from build123d import *

# Parameters (mm, degrees)
BOSS_EXTRUDE1_DEPTH      = 2
SKETCH3_R                = 0.5
CUT_EXTRUDE1_DEPTH       = 2
SKETCH4_R                = 0.75
BOSS_EXTRUDE2_DEPTH      = 1
SKETCH5_R                = 0.5
CUT_EXTRUDE2_DEPTH       = 2
BOSS_EXTRUDE3_DEPTH      = 3
BOSS_EXTRUDE3_DEPTH_BACK = 6
SKETCH6_R                = 2.5
SKETCH7_R                = 0.75
BOSS_EXTRUDE4_DEPTH      = 5
SKETCH9_R                = 0.65
BOSS_EXTRUDE5_DEPTH      = 0.3
BOSS_EXTRUDE6_DEPTH      = 2


with BuildPart() as part:
    # Sketch2 → Boss-Extrude1 (new body)
    with BuildSketch(Plane.XY):
        with BuildLine():
            Line((-7.9375, -2.462871108), (-7.9375, 2.462871108))
            ThreePointArc((-7.9375, 2.462871108), (-7.792847338, 2.889004109), (-7.418673332, 3.139019187))
            Line((-7.418673332, 3.139019187), (-0.924016143, 4.879257336))
            Line((-0.924016143, 4.879257336), (3.375983857, 4.879257336))
            ThreePointArc((3.375983857, 4.879257336), (3.870958604, 4.674232083), (4.075983857, 4.179257336))
            Line((4.075983857, 4.179257336), (4.075983857, 2.879257336))
            Line((4.075983857, 2.879257336), (7.075983857, 2.879257336))
            Line((7.075983857, 2.879257336), (7.075983857, 3.545029821))
            ThreePointArc((7.075983857, 3.545029821), (7.326032531, 4.081260931), (7.897537582, 4.234395248))
            Line((7.897537582, 4.234395248), (11.484053724, 3.601995685))
            ThreePointArc((11.484053724, 3.601995685), (11.89873111, 3.362581585), (12.0625, 2.912630258))
            Line((12.0625, 2.912630258), (12.0625, -2.912630258))
            ThreePointArc((12.0625, -2.912630258), (11.89873111, -3.362581585), (11.484053724, -3.601995685))
            Line((11.484053724, -3.601995685), (7.897537582, -4.234395248))
            ThreePointArc((7.897537582, -4.234395248), (7.326032531, -4.081260931), (7.075983857, -3.545029821))
            Line((7.075983857, -3.545029821), (7.075983857, -2.879257336))
            Line((7.075983857, -2.879257336), (4.075983857, -2.879257336))
            Line((4.075983857, -2.879257336), (4.075983857, -4.179257336))
            ThreePointArc((4.075983857, -4.179257336), (3.870958604, -4.674232083), (3.375983857, -4.879257336))
            Line((3.375983857, -4.879257336), (-0.924016143, -4.879257336))
            Line((-0.924016143, -4.879257336), (-7.418673332, -3.139019187))
            ThreePointArc((-7.418673332, -3.139019187), (-7.792847338, -2.889004109), (-7.9375, -2.462871108))
        make_face()
    extrude(amount=BOSS_EXTRUDE1_DEPTH)

    # Sketch3 → Cut-Extrude1 (cut)
    with BuildSketch(Plane.XY.offset(2)):
        with Locations((8.575983857, 2.879257336)):
            Circle(SKETCH3_R)
        with Locations((8.575983857, -2.879257336)):
            Circle(SKETCH3_R)
    extrude(amount=-CUT_EXTRUDE1_DEPTH, mode=Mode.SUBTRACT)

    # Sketch4 → Boss-Extrude2 (add)
    with BuildSketch(Plane.XY.offset(2)):
        with Locations((-7.9375, -1.7)):
            Circle(SKETCH4_R)
    extrude(amount=-BOSS_EXTRUDE2_DEPTH)

    # Sketch5 → Cut-Extrude2 (cut)
    with BuildSketch(Plane.XY.offset(2)):
        with Locations((-7.9375, -1.7)):
            Circle(SKETCH5_R)
    extrude(amount=-CUT_EXTRUDE2_DEPTH, mode=Mode.SUBTRACT)

    # Sketch6 → Boss-Extrude3 (add, two sides: drawn at the far end of the back side and taken through both)
    with BuildSketch(Plane.XY.offset(2).offset(-BOSS_EXTRUDE3_DEPTH_BACK)):
        Circle(SKETCH6_R)
    extrude(amount=BOSS_EXTRUDE3_DEPTH + BOSS_EXTRUDE3_DEPTH_BACK)

    # Sketch7 → Boss-Extrude4 (add)
    with BuildSketch(Plane.XY.offset(5)):
        Circle(SKETCH7_R)
    extrude(amount=BOSS_EXTRUDE4_DEPTH)

    # Sketch9 → Boss-Extrude5 (add)
    with BuildSketch(Plane.XY.offset(10)):
        Circle(SKETCH9_R)
    extrude(amount=BOSS_EXTRUDE5_DEPTH)

    # Sketch10 → Boss-Extrude6 (add)
    with BuildSketch(Plane.XY.offset(10.3)):
        with BuildLine():
            Line((0, 0.75), (0, -0.75))
            ThreePointArc((0, -0.75), (0.75, 0), (0, 0.75))
        make_face()
    extrude(amount=BOSS_EXTRUDE6_DEPTH)


solid = part.part
Model file for the job. Use its own axes, mm. A direction names the side the tool comes from. Round coordinates to 2 decimals unless told otherwise and drop trailing zeros. Order: outer loops, then holes, each group sorted by start corner. A loop starts at its lowest first (then second) coordinate and runs counter-clockwise, first axis right, second up. Notation, with made-up numbers: M 64.25,-16.75 L 89.25,-16.75 A25 cw 89.25,11.25 Z; hole C -30.75,15 d11. An arc over 180 degrees is marked long. Write each question's results on one line, items separated by ' | '. Start each with the question number.
(1) Saw through at A-A, the plane y = 0. Give the cut face in (x, z).
(2) Two-plate mould, pull along Y, no slides. Class faces 4 (the face through (1, -4.879, 1)), 5 (the face through (-7.46, -1.55, 1.24)), 6 (the face through (6, 2.879, 1)): pulls with the +Y half, pulls with the -Y half, needs draft (parallel to the pull), parting line crosses it, or undercut.
(3) Which spindle directions (+Z, -Z, +X, -X, +Y, -Y) get a long thin tool onto all of the face, cutting with end or side? Do faces 1 (the face through (2, 2, 0)), 2 (the face through (1, 1, 5)), 3 (the face through (4.076, -4, 1)). Say none if no direction does.
(4) Saw through at C-C, the plane x = 1.75. Give the cut face in (y, z), then the cut area to 3 significant figures.
(5) Saw through at B-B, the plane y = -1.7. Give the cut face in (x, z).
(6) Probe probe 1 along X at (y, z) = (-1.7, 1.1); probe 2 along Z at (x, y) = (1.75, -0.5); probe 3 along Z at (x, y) = (-4.25, 0.75). List the from-to ranges inside material, lowest first. Write a range as from..to.
(7) Saw through at D-D, the plane z = 3. Give the cut face in (x, y), then the cut area to 3 significant figures.
(8) Drop flat-ended pins along their axis: pin 1 (4 mm diameter, centred on x = -4, z = 2, fed in from +Y); pin 2 (0.6 mm diameter, centred on x = -8.5, y = -2, fed in from -Z); pin 3 (0.6 mm diameter, centred on y = 0.5, z = 1.5, fed in from -X). Give the stop position or say it passes through.
Established:
1) outline: M -7.94,0 L -2.5,0 L -2.5,-4 L 2.5,-4 L 2.5,0 L 12.06,0 L 12.06,2 L 2.5,2 L 2.5,5 L 0.75,5 L 0.75,10 L 0.65,10 L 0.65,10.3 L 0.75,10.3 L 0.75,12.3 L 0,12.3 L 0,10.3 L -0.65,10.3 L -0.65,10 L -0.75,10 L -0.75,5 L -2.5,5 L -2.5,2 L -7.94,2 Z
2) face 4: pulls with the -Y half | face 5: undercut | face 6: pulls with the +Y half
3) face 1: -Z | face 2: +Z | face 3: +Z, -Z, -Y
4) outline: M -4.88,0 L -1.79,0 L -1.79,-4 L 1.79,-4 L 1.79,0 L 4.88,0 L 4.88,2 L 1.79,2 L 1.79,5 L -1.79,5 L -1.79,2 L -4.88,2 Z | area: 44.5 mm^2
5) outline: M -8.69,1 L -8.44,1 L -8.44,2 L -8.69,2 Z; M -7.44,0 L -1.83,0 L -1.83,-4 L 1.83,-4 L 1.83,0 L 12.06,0 L 12.06,2 L 1.83,2 L 1.83,5 L -1.83,5 L -1.83,2 L -7.44,2 Z
6) probe 1: x = -8.69..-8.44, -7.44..12.06 | probe 2: z = -4..5 | probe 3: z = 0..2
7) outline: C 0,0 d5 | area: 19.6 mm^2
8) pin 1: stops at y = 4.59 | pin 2: stops at z = 1 | pin 3: stops at x = -7.94
